For this review, take the finished solid that the model builds, in its own axes (mm). A direction names the side the tool comes from. Coordinates: 2 decimals unless noted, no trailing zeros. Loops run counter-clockwise (first coordinate to the right, second up) from the corner with the lowest first, then second, coordinate; pieces in that order, holes last. Notation, with made-up numbers: (-22, -39.5) -> (18, -39.5) arc R19 ccw to (18, -18.5) -> close; hole circle Ø6 at (-36, -12.5). An arc over 180 degrees is marked (long way). Use a Markdown table: item, result.
from build123d import *

# Parameters (mm, degrees)
CUT_EXTRUDE1_DEPTH  = 172.877863613
SKETCH4_R           = 21
CUT_EXTRUDE3_DEPTH  = 161.832210704
SKETCH5_W           = 8
SKETCH5_H           = 3.5
BOSS_EXTRUDE1_DEPTH = 70
SKETCH6_R           = 15
CUT_EXTRUDE4_DEPTH  = 172.877863613
SKETCH7_W           = 8
SKETCH7_H           = 7
CUT_EXTRUDE5_DEPTH  = 172.877863613
SKETCH8_W           = 8
SKETCH8_H           = 0.543167705
BOSS_EXTRUDE2_DEPTH = 70


with BuildPart() as part:
    # Sketch1 → Revolve1 (revolve)
    with BuildSketch(Plane(origin=(0, 0, 0), x_dir=(1, 0, 0), z_dir=(0, 1, 0)), mode=Mode.PRIVATE) as revolve1_sk:
        with BuildLine():
            Line((0, 0), (0, 30))
            Line((0, 30), (35, 30))
            Line((35, 30), (35, 91))
            ThreePointArc((35, 91), (33.535533906, 94.535533906), (30, 96))
            Line((30, 96), (25, 96))
            Line((25, 96), (25, 111))
            Line((25, 111), (70, 111))
            Line((70, 111), (70, 0))
            Line((70, 0), (0, 0))
        make_face()
    revolve(revolve1_sk.sketch.rotate(Axis((-137.76, 0, 0), (1, 0, 0)), 180), axis=Axis((-137.76, 0, 0), (1, 0, 0)))

    # Sketch2 → Cut-Extrude1 (cut, through all)
    with BuildSketch(Plane.ZY):
        with BuildLine():
            Line((-4, 10.494049493), (-4, 17.494049493))
            Line((-4, 17.494049493), (4, 17.494049493))
            Line((4, 17.494049493), (4, 10.494049493))
            ThreePointArc((4, 10.494049493), (0, -11.230542051), (-4, 10.494049493))
        make_face()
    extrude(amount=-CUT_EXTRUDE1_DEPTH, mode=Mode.SUBTRACT)

    # Sketch4 → Cut-Extrude3 (cut, through all)
    with BuildSketch(Plane.ZY.offset(-35)):
        with Locations((0, 60)):
            Circle(SKETCH4_R)
        with Locations((51.961524227, 30)):
            Circle(SKETCH4_R)
        with Locations(Location((-51.961524227, 30, 0), (0, 0, 180))):
            Circle(SKETCH4_R)
        with Locations(Location((51.961524227, -30, 0), (0, 0, 180))):
            Circle(SKETCH4_R)
        with Locations(Location((0, -60, 0), (0, 0, 180))):
            Circle(SKETCH4_R)
        with Locations((-51.961524227, -30)):
            Circle(SKETCH4_R)
    extrude(amount=-CUT_EXTRUDE3_DEPTH, mode=Mode.SUBTRACT)

    # Sketch5 → Boss-Extrude1 (add)
    with BuildSketch(Plane.ZY):
        with Locations((0, 15.744049493)):
            Rectangle(SKETCH5_W, SKETCH5_H)
    extrude(amount=-BOSS_EXTRUDE1_DEPTH)

    # Sketch6 → Cut-Extrude4 (cut, through all)
    with BuildSketch(Plane.ZY):
        Circle(SKETCH6_R)
    extrude(amount=-CUT_EXTRUDE4_DEPTH, mode=Mode.SUBTRACT)

    # Sketch7 → Cut-Extrude5 (cut, through all)
    with BuildSketch(Plane.ZY):
        with Locations((0, 15)):
            Rectangle(SKETCH7_W, SKETCH7_H)
    extrude(amount=-CUT_EXTRUDE5_DEPTH, mode=Mode.SUBTRACT)

    # Sketch8 → Boss-Extrude2 (add)
    with BuildSketch(Plane.ZY):
        with Locations((0, 18.228416147)):
            Rectangle(SKETCH8_W, SKETCH8_H)
    extrude(amount=-BOSS_EXTRUDE2_DEPTH)


solid = part.part
(1) Mouldability with a two-part tool opening along Z and no side actions: class faces 4 (the face through (25, -83, 50)), 5 (the face through (17.745, -25.296, 16.128)), 6 (the face through (47.815, -33.341, 105.874)), 7 (the face through (35, -21.5, 21.5)) as pulls with the +Z half, pulls with the -Z half, needs draft (parallel to the pull), parting line crosses it, or undercut.
Found:
| item | result |
|---|---|
| face 4 | needs draft |
| face 5 | undercut |
| face 6 | parting line crosses it |
| face 7 | undercut |
(2) For pin 1 Ø1 at (x, y) = (43.5, 17) entering from +Z; pin 2 Ø12 at (x, z) = (37.5, 24.5) entering from -Y; pin 3 Ø6 at (y, z) = (-34, -0.5) entering from -X, all flat-tipped, find the tip position at first contact; note any pin that passes through.
Found:
| item | result |
|---|---|
| pin 1 | stops at z = 109.77 |
| pin 2 | stops at y = -109.45 |
| pin 3 | stops at x = 35 |
(3) Take a section at C-C on x = 52. Write out the cut boundary in (y, z).
Found:
| item | result |
|---|---|
| outline | circle Ø222 at (0, 0); hole circle Ø42 at (-60, 0); hole circle Ø42 at (-30, -51.96); hole circle Ø42 at (-30, 51.96); hole circle Ø42 at (30, -51.96); hole circle Ø42 at (30, 51.96); hole (14.46, -4) -> (17.96, -4) -> (17.96, 4) -> (14.46, 4) arc R15 ccw (long way) to start; hole circle Ø42 at (60, 0) |
(4) Take a section at A-A on x = 15. Write out the cut boundary in (y, z), plus the area to 3 significant figures.
Found:
| item | result |
|---|---|
| outline | circle Ø60 at (0, 0); hole (14.46, -4) -> (17.96, -4) -> (17.96, 4) -> (14.46, 4) arc R15 ccw (long way) to start |
| area | 2,100 mm^2 |
(5) Take a section at B-B on y = 0. Write out the cut boundary in (x, z).
Found:
| item | result |
|---|---|
| outline | (0, -30) -> (35, -30) -> (35, -91) arc R5 cw to (30, -96) -> (25, -96) -> (25, -111) -> (70, -111) -> (70, -15) -> (0, -15) -> close; (0, 15) -> (70, 15) -> (70, 111) -> (25, 111) -> (25, 96) -> (30, 96) arc R5 cw to (35, 91) -> (35, 30) -> (0, 30) -> close |
(6) For faces 1 (the face through (27.465, -28.836, 91.567)), 2 (the face through (0, 14, 6)), 3 (the face through (35, 17.957, 0)), list the 3-axis set-ups (+Z, -Z, +X, -X, +Y, -Y) from which the entire face can be reached by the end or side of a thin tool; tool diameter is ignored.
Found:
| item | result |
|---|---|
| face 1 | -X |
| face 2 | +Z, -Z, -X, +Y, -Y |
| face 3 | +X, -X |
(7) Take a section at D-D on z = 62.5. State how many separate pieces and enclosed holes the cut face has, plus the area to 3 significant figures.
Found:
| item | result |
|---|---|
| separate pieces | 3 |
| enclosed holes | 0 |
| area | 4,270 mm^2 |
(8) For line 1 along Y through (x, z) = (55.5, 0); line 2 along Y through (x, z) = (44, -18.5); line 3 along Z through (x, y) = (39, -43), list the stretches that pass through material, from the lowest coordinate up.
Found:
| item | result |
|---|---|
| line 1 | y = -111 to -81, -39 to -15, 17.96 to 39, 81 to 111 |
| line 2 | y = -109.45 to -69.94, -50.06 to 50.06, 69.94 to 109.45 |
| line 3 | z = -102.33 to -68.45, -35.47 to -12.33, 12.33 to 35.47, 68.45 to 102.33 |
